Could you check a few things on this model? Use its own coordinates, in mm. Coordinates: 2 decimals unless noted, no trailing zeros. Write each loop counter-clockwise with the first axis right and the second up, starting at its lowest first coordinate (ties: lowest second). Pieces come first, ordered by that corner, then holes.
Item 1: I want a section at D-D on x = -7.5. Please give me the cut outline in (y, z), then the cut area to 3 significant figures.
Item 2: I want a section at C-C on y = 0. Please give me the cut outline in (x, z).
Item 3: Thinking about a two-plate mould opening in X: for faces 1 (the flat face through (-15.868, -7, 6)), 2 (the cylindrical face through (4.727, 6.822, 4.334)), 3 (the flat face through (3, 2, 0)), 4 (the cylindrical face through (-7.04, 6.84, 6.26)), which applies, +X half, -X half, draft (parallel to the pull), parting line (faces both ways), or undercut?
Item 4: If I drill on probe 1 along Y at (x, z) = (-11.5, 4); probe 2 along X at (y, z) = (-19, 10.25); probe 3 along Y at (x, z) = (-7.5, 3.5), over which ranges is the centre line in solid material (lowest first)?
Item 5: I want a section at B-B on z = 6.5. Please give me the cut outline in (x, y).
Item 6: I want a section at A-A on y = -21. Please give me the cut outline in (x, z).
Autodesk Inventor part; units mm, degrees
ref_plane "YZ Plane" through (0, 0, 0) normal (1, 0, 0) x (0, 1, 0)
ref_plane "XZ Plane" through (0, 0, 0) normal (0, 1, 0) x (-1, 0, 0)
ref_plane "XY Plane" through (0, 0, 0) normal (0, 0, 1) x (1, 0, 0)
sketch "Sketch1" plane through (0, 0, 0) normal (0, 0, 1) x (1, 0, 0)
  line L0 (-15.8683, 12.6347) -> (22.2317, 12.6347)
  line L1 (22.2317, 12.6347) -> (22.2317, -25.4653)
  line L2 (22.2317, -25.4653) -> (-15.8683, -25.4653)
  line L3 (-15.8683, -25.4653) -> (-15.8683, 12.6347)
  point P0 (0, 0)
  dimension "d0" = 38.1
  dimension "d1" = 38.1
extrude "Extrusion1" add sketch "Sketch1" along normal blind 12.7
hole "Hole1" at (3.1817, -6.4153, 12.7) direction (0, 0, -1) diameter 16 end through all
hole "Hole2" at (-9.5183, 6.2847, 12.7) direction (0, 0, -1) diameter 5.08 end through all
hole "Hole3" at (15.8817, 6.2847, 12.7) direction (0, 0, -1) diameter 5.08 end through all
hole "Hole4" at (-9.5183, -19.1153, 12.7) direction (0, 0, -1) diameter 5.08 end through all
hole "Hole5" at (15.8817, -19.1153, 12.7) direction (0, 0, -1) diameter 5.08 end through all
hole "Hole6" at (3.1817, 12.6347, 6.35) direction (0, -1, 0) diameter 5.08 depth 12.7 tip angle 118
sketch "Sketch2" plane through (0, 0, 12.7) normal (0, 0, 1) x (1, 0, 0)
  circle A0 centre (15.8817, -19.1153) radius 2.54
  circle A1 centre (-9.5183, -19.1153) radius 2.54
  circle A2 centre (15.8817, 6.2847) radius 2.54
  circle A3 centre (-9.5183, 6.2847) radius 2.54
  circle A4 centre (3.1817, -6.4153) radius 8
  line L0 (22.2317, 12.6347) -> (22.2317, -25.4653)
  line L1 (-15.8683, 12.6347) -> (22.2317, 12.6347)
  line L2 (-15.8683, -25.4653) -> (-15.8683, 12.6347)
  line L3 (22.2317, -25.4653) -> (-15.8683, -25.4653)
  point P0 (0, 0)
  dimension "d58" = 6.35
  dimension "d59" = 6.35
  dimension "d60" = 19.05
  dimension "d61" = 19.05
  dimension "d64" = 16
  dimension "d65" = 12.7
  dimension "d66" = 12.7
  dimension "d67" = 12.7
sketch "Sketch3" plane through (-15.8683, 12.6347, 0) normal (0, 1, 0) x (1, 0, 0)
  circle A0 centre (19.05, -6.35) radius 2.54
  line L0 (0, -12.7) -> (38.1, -12.7)
  line L1 (38.1, 0) -> (38.1, -12.7)
  line L2 (0, 0) -> (38.1, 0)
  line L3 (0, 0) -> (0, -12.7)
  point P0 (15.8683, 0)
  dimension "d62" = 6.35
  dimension "d63" = 19.05
properties part number "alignmentplate"
Response values:
1. outline: (-25.47, 0) - (-20.66, 0) - (-20.66, 12.7) - (-25.47, 12.7) - close; (-17.57, 0) - (4.74, 0) - (4.74, 12.7) - (-17.57, 12.7) - close; (7.83, 0) - (12.63, 0) - (12.63, 12.7) - (7.83, 12.7) - close
1. area: 406 mm2
2. outline: (-15.87, 0) - (-1.6, 0) - (-1.6, 12.7) - (-15.87, 12.7) - close; (7.96, 0) - (22.23, 0) - (22.23, 12.7) - (7.96, 12.7) - close
3. face 1: -X half
3. face 2: undercut
3. face 3: draft
3. face 4: undercut
4. probe 1: y = -25.47 to -20.7, -17.53 to 4.7, 7.87 to 12.63
4. probe 2: x = -15.87 to -12.06, -6.98 to 13.34, 18.42 to 22.23
4. probe 3: y = -25.47 to -20.66, -17.57 to 4.74, 7.83 to 12.63
5. outline: (-15.87, -25.47) - (22.23, -25.47) - (22.23, 12.63) - (5.72, 12.63) - (5.72, 1.17) arc R8 cw (long way) to (0.65, 1.17) - (0.65, 12.63) - (-15.87, 12.63) - close; hole circle Ø5.08 at (-9.52, -19.12); hole circle Ø5.08 at (-9.52, 6.28); hole circle Ø5.08 at (15.88, -19.12); hole circle Ø5.08 at (15.88, 6.28)
6. outline: (-15.87, 0) - (-11.22, 0) - (-11.22, 12.7) - (-15.87, 12.7) - close; (-7.82, 0) - (14.18, 0) - (14.18, 12.7) - (-7.82, 12.7) - close; (17.58, 0) - (22.23, 0) - (22.23, 12.7) - (17.58, 12.7) - close
